Study the drawing (mm; zero at the part's minimum x, y, z) and answer. A direction names the side the tool comes from. Coordinates: 2 decimals unless noted, no trailing zeros. Loops run counter-clockwise (first coordinate to the right, second up) from the corner with the lowest first, then second, coordinate; pieces in that order, holes last. Notation, with made-up numbers: (67.5, 76) -> (93.5, 76) arc R16 cw to (93.5, 104) -> close; hole circle Ø6 at (61.25, -37.5). An arc over 180 degrees is marked (long way). One line per question, with ' | ' between items. Start each with the question number.
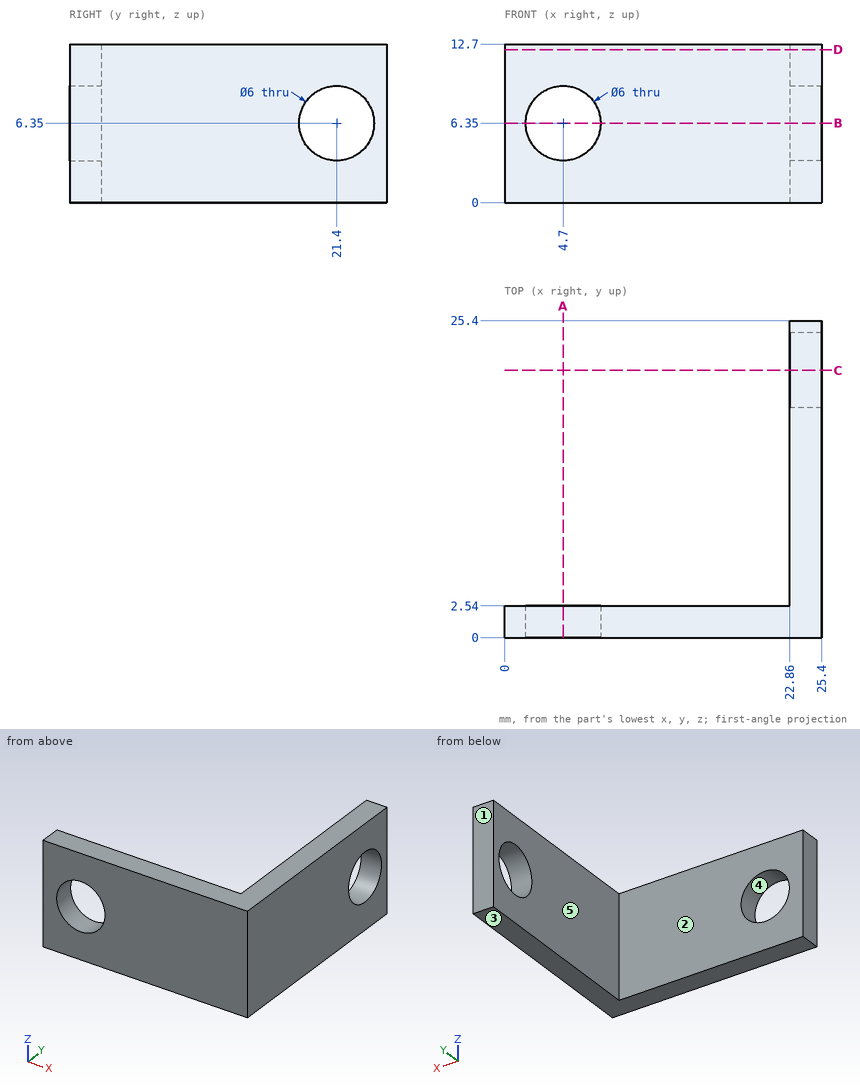
(1) Section A-A on x = 4.7 is taken. Write down the section's boundary in (y, z).
(2) Section B-B on z = 6.35 is taken. Write down the section's boundary in (x, y).
(3) Section D-D on z = 12.25 is taken. Write down the section's boundary in (x, y).
(4) Section C-C on y = 21.4 is taken. Write down the section's boundary in (x, z), plus the area to 3 significant figures.
(5) Determine the mould class of the marked faces 3, 4 and 5 for opening direction X: +X half, -X half, draft (parallel to the pull), parting line (faces both ways), or undercut.
(6) A tool of negligible diameter and unlimited length cuts with its end or side. For the marked faces 1 and 2, from which of +Z, -Z, +X, -X, +Y, -Y can it reach the whole face along a straight path? Write none if from no direction.
(7) Each of these flat-tipped pins is pushed along its axis until it touches: pin 1 Ø4 at (y, z) = (19, 11) entering from -X; pin 2 Ø6.5 at (x, z) = (17, 9) entering from +Y. Where does it stop, or does it pass through?
(8) Find the intervals of material crossed by probe 1 along Y at (x, z) = (23.4, 6.35); probe 2 along Y at (x, z) = (6.5, 2.75); probe 3 along Z at (x, y) = (4.7, 1), in increasing order. Write a range as from..to.
Working result:
1) outline: (0, 0) -> (2.54, 0) -> (2.54, 3.35) -> (0, 3.35) -> close; (0, 9.35) -> (2.54, 9.35) -> (2.54, 12.7) -> (0, 12.7) -> close
2) outline: (0, 0) -> (1.7, 0) -> (1.7, 2.54) -> (0, 2.54) -> close; (7.7, 0) -> (25.4, 0) -> (25.4, 18.4) -> (22.86, 18.4) -> (22.86, 2.54) -> (7.7, 2.54) -> close; (22.86, 24.4) -> (25.4, 24.4) -> (25.4, 25.4) -> (22.86, 25.4) -> close
3) outline: (0, 0) -> (25.4, 0) -> (25.4, 25.4) -> (22.86, 25.4) -> (22.86, 2.54) -> (0, 2.54) -> close
4) outline: (22.86, 0) -> (25.4, 0) -> (25.4, 3.35) -> (22.86, 3.35) -> close; (22.86, 9.35) -> (25.4, 9.35) -> (25.4, 12.7) -> (22.86, 12.7) -> close | area: 17.0 mm2
5) face 3: draft | face 4: undercut | face 5: -X half
6) face 1: +Z, -Z, +X, -X, +Y | face 2: +Z, -Z, -X, +Y
7) pin 1: stops at x = 22.86 | pin 2: stops at y = 2.54
8) probe 1: y = 0..18.4, 24.4..25.4 | probe 2: y = 0..2.54 | probe 3: z = 0..3.35, 9.35..12.7
